Autodesk Inventor part; units mm, degrees
ref_plane "YZ Plane" through (0, 0, 0) normal (1, 0, 0) x (0, 1, 0)
ref_plane "XZ Plane" through (0, 0, 0) normal (0, 1, 0) x (-1, 0, 0)
ref_plane "XY Plane" through (0, 0, 0) normal (0, 0, 1) x (1, 0, 0)
sketch "Sketch1" plane through (0, 0, 0) normal (0, 0, 1) x (1, 0, 0)
  line L0 (0, 0) -> (50, 0)
  line L1 (50, 0) -> (50, 50)
  line L2 (50, 50) -> (0, 50)
  line L3 (0, 50) -> (0, 0)
  dimension "d0" = 50
  dimension "d1" = 50
extrude "Extrusion1" add sketch "Sketch1" along normal blind 40
sketch "Sketch2" plane through (0, 0, 40) normal (0, 0, 1) x (1, 0, 0)
  line L0 (50, 0) -> (50, 50)
  line L1 (50, 15) -> (9, 15)
  line L2 (9, 15) -> (9, 35)
  line L3 (9, 35) -> (50, 35)
  line L4 (50, 35) -> (50, 15)
  line L5 (0, 0) -> (50, 0)
  point P0 (50, 35)
  dimension "d4" = 41
  dimension "d5" = 20
  dimension "d6" = 15
extrude "Extrusion2" cut sketch "Sketch2" against normal blind 17.5
sketch "Sketch3" plane through (0, 0, 0) normal (-1, 0, 0) x (0, 0, 1)
  line L0 (40, 50) -> (40, 0)
  line L1 (40, 35) -> (18.5, 35) construction
  line L2 (40, 35) -> (61.5, 35) construction
  line L3 (18.5, 35) -> (18.5, 15) construction
  line L4 (18.5, 15) -> (40, 15) construction
  line L5 (0, 50) -> (40, 50)
  line L6 (40, 29.85) -> (18.5, 29.85) construction
  line L7 (40, 20.15) -> (18.5, 20.15) construction
  point P0 (0, 0)
  dimension "d9" = 21.5
  dimension "d10" = 180
  dimension "d11" = 20
  dimension "d12" = 15
  dimension "d13" = 5.15
  dimension "d14" = 5.15
hole "Hole1" at (0, 29.85, 18.5) at (0, 20.15, 18.5) direction (1, 0, 0) diameter 4.3 end through all
sketch "Sketch4" plane through (0, 0, 22.5) normal (0, 0, 1) x (1, 0, 0)
  line L0 (9, 35) -> (50, 35)
  line L1 (50, 15) -> (9, 15)
  line L2 (18, 35) -> (20.4, 35)
  line L3 (20.4, 35) -> (20.4, 15)
  line L4 (20.4, 15) -> (18, 15)
  line L5 (18, 15) -> (18, 35)
  line L6 (9, 15) -> (9, 35)
  point P0 (0, 0)
  point P1 (18, 15)
  dimension "d22" = 9
  dimension "d23" = 2.4
extrude "Extrusion3" cut sketch "Sketch4" against normal blind 7 contours L0 L3 L1 L5
chamfer "Chamfer1" distance 5 angle 45 4 edges at (0, 50, 20) (50, 50, 20) (0, 0, 20) (50, 0, 20)
sketch "Sketch7" plane through (0, 0, 22.5) normal (0, 0, 1) x (1, 0, 0)
  line L0 (18, 15) -> (18, 35)
  line L1 (18, 24.5) -> (16, 24.5)
  line L2 (16, 24.5) -> (16, 25.5)
  line L3 (16, 25.5) -> (18, 25.5)
  line L4 (18, 25.5) -> (18, 24.5)
  line L5 (9, 35) -> (50, 35)
  point P0 (0, 0)
  dimension "d45" = 2
  dimension "d46" = 1
  dimension "d47" = 9.5
extrude "Extrusion5" cut sketch "Sketch7" against normal blind 7
chamfer "Chamfer3" distance 7 distance2 2 1 edges at (16, 25, 15.5) measured on face at (16, 25.1667, 20.1667)
sketch "Sketch8" plane through (0, 0, 0) normal (0, 0, -1) x (-1, 0, 0)
  line L0 (-5, 0) -> (-45, 0)
  line L1 (-14.2086, 0) -> (-34.2086, 0)
  line L2 (-34.2086, 0) -> (-34.2086, 7.5)
  line L3 (-34.2086, 7.5) -> (-14.2086, 7.5)
  line L4 (-14.2086, 7.5) -> (-14.2086, 0)
  point P0 (0, 0)
  dimension "d53" = 20
  dimension "d54" = 7.5
extrude "Extrusion6" add sketch "Sketch8" along normal blind 30
fillet "Fillet2" radius 10 2 edges at (34.2086, 3.75, -30) (14.2086, 3.75, -30)
chamfer "Chamfer4" distance 3 angle 45 2 edges at (34.2086, 3.75, 0) (14.2086, 3.75, 0)
sketch "Sketch9" plane through (24.2086, 7.5, -20) normal (0, 1, 0) x (1, 0, 0)
  line L0 (13, -20) -> (-13, -20)
  line L1 (0, -20) -> (0, 0) construction
  point P0 (-24.2086, -20)
  dimension "d61" = 20
hole "Hole3" at (24.2086, 7.5, -20) direction (0, -1, 0) diameter 5 end through all counterbore diameter 6 counterbore depth 4
properties part number "ES117_MP1"
Source: CAD feature listing. Evaluate the final solid. Frame: model axes, mm. A direction names the side the tool comes from. Give positions to 0.01 mm unless a question says otherwise; leave off trailing zeros. Write each loop counter-clockwise with the first axis right and the second up, starting at its lowest first coordinate (ties: lowest second). Pieces come first, ordered by that corner, then holes.
1. Material intervals for line 1 along Y through (x, z) = (11.5, 28.5); line 2 along X through (y, z) = (17.5, 16); line 3 along Y through (x, z) = (22, -25.5), sorted ascending.
2. Section query C-C (z = 18.5). Count the separate pieces of the cut face and the enclosed holes in it, then the cut area to 3 significant figures.
3. Access query for faces 1 (the face through (34.209, 4, -11)), 2 (the face through (14.209, 4, -11)), 3 (the face through (35, 25, 22.5)), 4 (the face through (24, 7.5, -15)), 5 (the face through (20.4, 25, 19)). Directions: +Z, -Z, +X, -X, +Y, -Y. A direction counts if a zero-diameter tool reaches every point of the face in a straight line with its end or side. Return the directions, or none.
4. Section query A-A (y = 20.15). Return the cut outline in (x, z), then the cut area to 3 significant figures.
5. Section query B-B (x = 44). Return the cut outline in (y, z), then the cut area to 3 significant figures.
6. Section query D-D (z = 8). Return the cut outline in (x, y).
7. Pull-direction query (Z, two-part tool) for faces 6 (the face through (9, 25, 31)), 7 (the face through (9.13, 18.02, 18.22)), 8 (the face through (17, 25, 19)), 9 (the face through (25, 25, 0)); classes: +Z half, -Z half, draft (parallel to the pull), parting line (faces both ways), or undercut.
8. First-contact query: pin 1 (2 mm diameter, centred on y = 3, z = -10, fed in from -X); pin 2 (5 mm diameter, centred on y = 29, z = 33, fed in from +X); pin 3 (0.7 mm diameter, centred on x = 19.5, y = 26.5, fed in from +Z); pin 4 (4 mm diameter, centred on y = 29.85, z = 18.5, fed in from -X). Flat tips, straight axial feed; report the tip coordinate or a pass-through.
Output values:
1. line 1: y = 0 to 15, 35 to 50
1. line 2: x = 0 to 18, 20.4 to 50
1. line 3: y = 0 to 7.5
2. separate pieces: 4
2. enclosed holes: 0
2. area: 1,990 mm2
3. face 1: -Z, +X, +Y, -Y
3. face 2: -Z, -X, +Y, -Y
3. face 3: +Z, +X
3. face 4: -Z, +X, -X, +Y
3. face 5: +Z
4. outline: (0, 0) - (50, 0) - (50, 16.35) - (20.4, 16.35) - (20.4, 15.5) - (18, 15.5) - (18, 16.35) - (0, 16.35) - close; (0, 20.65) - (18, 20.65) - (18, 22.5) - (9, 22.5) - (9, 40) - (0, 40) - close; (20.4, 20.65) - (50, 20.65) - (50, 22.5) - (20.4, 22.5) - close
4. area: 1,060 mm2
5. outline: (0, 0) - (50, 0) - (50, 40) - (35, 40) - (35, 22.5) - (15, 22.5) - (15, 40) - (0, 40) - close; hole circle Ø4.3 at (20.15, 18.5); hole circle Ø4.3 at (29.85, 18.5)
5. area: 1,620 mm2
6. outline: (0, 5) - (5, 0) - (45, 0) - (50, 5) - (50, 45) - (45, 50) - (5, 50) - (0, 45) - close
7. face 6: draft
7. face 7: undercut
7. face 8: +Z half
7. face 9: -Z half
8. pin 1: stops at x = 14.21
8. pin 2: stops at x = 9
8. pin 3: stops at z = 15.5
8. pin 4: passes through
